from build123d import *

# Parameters (mm, degrees)
F1_DEPTH = 16
F2_W     = 10
F2_H     = 2
F3_DEPTH = 9.906
F2_W_2   = 9.277396
F2_H_2   = 2.0066
F4_DEPTH = 9.652
F5_R     = 2.5
F6_DEPTH = 17.5006


with BuildPart() as f1:
    # F0 (on Front) → F1 (new body)
    with BuildSketch(Plane.XZ):
        Polygon((-25, 0), (0, 0), (0, 20), (-25, 31.029411), align=None)
    extrude(amount=F1_DEPTH)

    # F2 (on face) → F3 (join)
    with BuildSketch(Plane(origin=(7.385952, 0, 16.741492), x_dir=(0.914918, 0, -0.40364), z_dir=(0.40364, 0, 0.914918))):
        with Locations((-21.735233, -3)):
            Rectangle(F2_W, F2_H)
    extrude(amount=F3_DEPTH)

    # F2 (on face) → F4 (join)
    with BuildSketch(Plane(origin=(7.385952, 0, 16.741492), x_dir=(0.914918, 0, -0.40364), z_dir=(0.40364, 0, 0.914918))):
        with Locations((-21.735233, -3)):
            Rectangle(F2_W, F2_H)
        with Locations((-21.370131, -12.9967)):
            Rectangle(F2_W_2, F2_H_2)
    extrude(amount=F4_DEPTH)

    # F5 (on face) → F6 (cut)
    with BuildSketch(Plane(origin=(0, -2, 0), x_dir=(-1, 0, 0), z_dir=(0, 1, 0))):
        with Locations((10.50077, 30.046294)):
            Circle(F5_R)
    extrude(amount=-F6_DEPTH, mode=Mode.SUBTRACT)


solid = f1.part
Model file for the job. Use its own axes, mm. A direction names the side the tool comes from. Give positions to 0.01 mm unless a question says otherwise; leave off trailing zeros. Order: outer loops, then holes, each group sorted by start corner. A loop starts at its lowest first (then second) coordinate and runs counter-clockwise, first axis right, second up. Notation, with made-up numbers: M 62,87.5 L 75,87.5 A15 cw 75,111.5 Z; hole C 69,36.25 d5. An arc over 180 degrees is marked long. Put each result on its own line as item: value. Start each with the question number.
(1) Band-saw the part on B-B on y = -13.25. Give the cut face in (x, z), then the cut area to 3 significant figures.
(2) Band-saw the part on D-D on z = 21.5. Give the cut face in (x, y).
(3) Band-saw the part on C-C on y = -5. Give the cut face in (x, z), then the cut area to 3 significant figures.
(4) Pin check, flat tips, straight feed: pin 1 Ø3 at (x, z) = (-10.5, 30.05) entering from +Y; pin 2 Ø1.5 at (x, y) = (-19.5, -9) entering from +Z; pin 3 Ø2 at (y, z) = (-13, 26) entering from +X; pin 4 Ø3.5 at (x, z) = (-13, 30) entering from -Y. Stop position of each tip, or through.
(5) Drill centre lines: L1, parallel to Y at x = -13.75, z = 30; L2, parallel to Z at x = -9, y = -13.25; L3, parallel to Z at x = -20.25, y = -14. Where is each one in solid material? Low to high. Write a range as [from, to].
(6) Pull direction Y, two halves, no side cores. Call faces 1 (the face through (-8.9, -11.993, 27.9)), 2 (the face through (-13, 0, 12)), 3 (the face through (-8.57, -2.99, 34.61)): released by +Y, released by -Y, zero draft, split by the parting line, or undercut.
(7) Band-saw the part on A-A on x = -11.5. Give the cut face in (y, z).
(8) Tool access for faces 4 (the face through (-14, -4, 29)), 5 (the face through (-6, -13.01, 27.85)), 6 (the face through (-8.9, -14, 27.9)), 7 (the face through (-15.103, -3.014, 32.001)), 8 (the face through (-14, -2, 29)): list every direction of +Z, -Z, +X, -X, +Y, -Y with a clear straight run to the whole face (end or side of a thin tool).
Results below:
1. outline: M -25,0 L 0,0 L 0,20 L -7.92,23.49 L -4.03,32.33 L -12.51,36.07 L -16.41,27.24 L -25,31.03 Z; hole C -10.5,30.05 d5
1. area: 708 mm2
2. outline: M -25,-16 L -3.4,-16 L -3.4,0 L -25,0 Z
3. outline: M -25,0 L 0,0 L 0,20 L -25,31.03 Z
3. area: 638 mm2
4. pin 1: passes through
4. pin 2: stops at z = 28.93
4. pin 3: stops at x = -6.38
4. pin 4: stops at y = -14
5. L1: y = [-14, -11.99], [-4, -2]
5. L2: z = [0, 28.05], [32.05, 34.52]
5. L3: z = [0, 28.93]
6. face 1: undercut
6. face 2: released by +Y
6. face 3: zero draft
7. outline: M -16,0 L 0,0 L 0,25.07 L -2,25.07 L -2,27.75 L -4,27.75 L -4,25.07 L -11.99,25.07 L -11.99,27.75 L -14,27.75 L -14,25.07 L -16,25.07 Z; M -14,32.34 L -11.99,32.34 L -11.99,35.62 L -14,35.62 Z; M -4,32.34 L -2,32.34 L -2,35.9 L -4,35.9 Z
8. face 4: +Z, +X
8. face 5: +X, +Y, -Y
8. face 6: +Z, +X, -Y
8. face 7: +Z, +Y, -Y
8. face 8: +Z, +X, +Y
